Geometry: final body of the model. Coordinates: model frame, mm. A direction names the side the tool comes from. Give positions to 0.01 mm unless a question says otherwise; leave off trailing zeros. Write each loop counter-clockwise with the first axis right and the second up, starting at its lowest first coordinate (ties: lowest second). Pieces come first, ordered by that corner, then holes. Notation, with made-up numbers: M 12.25,57 L 36.25,57 A21 cw 36.25,87 Z; hole C -27.75,-4 d8. An arc over 180 degrees is marked long. Use a Markdown table: item, result. Add a question column.
(1) Material intervals for L1, parallel to Y at x = 0.25, z = -42.5; L2, parallel to X at y = -1.75, z = 6.5; L3, parallel to X at y = -6, z = -11, sorted ascending.
(2) Cut plane B-B (z = -25). Output: boundary loops of the cut face in (x, y), plus the area to 3 significant figures.
(3) Draft query along Z for faces 3 (the conical face through (1.55, 4.93, 40.47)), 4 (the flat face through (6, 0, 50)), 5 (the flat face through (0, 0, -50)). Return one class per face: released by +Z, released by -Z, zero draft, split by the parting line, or undercut.
(4) Pin query (flat end, axial travel): pin 1 Ø8 at (y, z) = (-5, -6) entering from -X; pin 2 Ø2 at (x, z) = (-2.5, -30.5) entering from -Y; pin 3 Ø4 at (y, z) = (0, 49) entering from -X. Return the tip coordinate at first contact, or that it passes through.
(5) Cut plane A-A (y = 0). Output: boundary loops of the cut face in (x, z), plus the area to 3 significant figures.
(6) Reachability of faces 1 (the flat face through (-6, 0, 50)), 2 (the cylindrical face through (-7.81, -1.73, -9.44)) from +Z, -Z, +X, -X, +Y, -Y: full face, straight path, thin tool, end or side. Return the list, or none.
```python
from build123d import *

# Parameters (mm, degrees)
SKETCH3_R                = 2.5
BOSS_EXTRUDE1_DEPTH      = 6
BOSS_EXTRUDE1_DEPTH_BACK = 6


with BuildPart() as part:
    # Sketch2 → Revolve1 (revolve)
    with BuildSketch(Plane(origin=(0, 0, 0), x_dir=(0, 0, -1), z_dir=(1, 0, 0))):
        with BuildLine():
            Line((50, 0), (50, 8))
            Line((50, 8), (-30, 8))
            Line((-30, 8), (-50.652805728, 2.413264321))
            ThreePointArc((-50.652805728, 2.413264321), (-51.985197008, 1.519537048), (-52.5, 0))
            Line((-52.5, 0), (50, 0))
        make_face()
    revolve(axis=Axis((0, 0, 50), (0, 0, -1)))

    # Sketch3 → Boss-Extrude1 (add, two sides)
    with BuildSketch(Plane(origin=(0, 0, 0), x_dir=(0, 0, -1), z_dir=(1, 0, 0))) as boss_extrude1_sk:
        with Locations((-50, 0)):
            Circle(SKETCH3_R)
    extrude(amount=BOSS_EXTRUDE1_DEPTH)
    extrude(boss_extrude1_sk.sketch, amount=-BOSS_EXTRUDE1_DEPTH_BACK)


solid = part.part
```
Answer list:
| question | item | result |
|---|---|---|
| 1 | L1 | -8 to 8 |
| 1 | L2 | -7.81 to 7.81 |
| 1 | L3 | -5.29 to 5.29 |
| 2 | outline | C 0,0 d16 |
| 2 | area | 201 mm² |
| 3 | face 3 | undercut |
| 3 | face 4 | zero draft |
| 3 | face 5 | released by -Z |
| 4 | pin 1 | x = -7.94 |
| 4 | pin 2 | y = -7.86 |
| 4 | pin 3 | x = -6 |
| 5 | outline | M -8,-50 L 8,-50 L 8,30 L 3.27,47.5 L 6,47.5 L 6,52.5 L -6,52.5 L -6,47.5 L -3.27,47.5 L -8,30 Z |
| 5 | area | 1,540 mm² |
| 6 | face 1 | +Z, -X, +Y, -Y |
| 6 | face 2 | +Z, -Z |
